Design review of the part built by this model. Coordinates are the model's own, in mm. Face numbers are marked on the shaded views. A direction names the side the tool comes from. Give positions to 0.01 mm unless a question says otherwise; leave off trailing zeros. Loops run counter-clockwise (first coordinate to the right, second up) from the corner with the lowest first, then second, coordinate; pieces in that order, holes last. Notation, with made-up numbers: M 8.25,8.25 L 39.25,8.25 A18 cw 39.25,34.25 Z; hole C 80,68 d7. An arc over 180 degrees is marked long. Use CSV: the item, a comma, the result in double quotes.
from build123d import *

# Parameters (mm, degrees)
F1_DEPTH = 31.75
F3_DEPTH = 2.032
F4_SIZE  = 5.08
F5_R     = 3.175
F6_DEPTH = 3.048
F7_R     = 1.5875
F9_DEPTH = 22.0939118459


with BuildPart() as f1:
    # F0 (on Top) → F1 (new body)
    with BuildSketch(Plane.XY):
        Polygon((-25.273, 19.05), (-25.273, 0), (25.273, 0), (25.273, 19.05), (44.45, 19.05), (44.45, 22.098), (22.225, 22.098), (22.225, 3.048), (-22.225, 3.048), (-22.225, 22.098), (-44.45, 22.098), (-44.45, 19.05), align=None)
    extrude(amount=F1_DEPTH)

    # F2 (on face) → F3 (join)
    with BuildSketch(Plane(origin=(0, 0, 0), x_dir=(1, 0, 0), z_dir=(0, 0, -1))):
        Polygon((25.273, 0), (-25.273, 0), (-25.273, -19.05), (-44.45, -19.05), (-44.45, -22.098), (-25.273, -22.098), (-6.35, -22.098), (-6.35, -18.923), (6.35, -18.923), (6.35, -22.098), (25.273, -22.098), (44.45, -22.098), (44.45, -19.05), (25.273, -19.05), align=None)
    extrude(amount=F3_DEPTH)

    # F4
    f4_edges = [f1.edges().sort_by_distance(p)[0] for p in [
        (44.45, 20.574, 31.75),
        (-44.45, 20.574, 31.75),
    ]]
    chamfer(f4_edges, length=F4_SIZE)

    # F5 (on face) → F6 (cut, through all)
    with BuildSketch(Plane.XZ.offset(-19.05)):
        with Locations((-34.8615, 12.319)):
            Circle(F5_R)
        with Locations((34.8615, 12.319)):
            Circle(F5_R)
    extrude(amount=-F6_DEPTH, mode=Mode.SUBTRACT)

    # F7
    f7_edges = [f1.edges().sort_by_distance(p)[0] for p in [
        (25.273, 0, 14.859),
        (-25.273, 0, 14.859),
        (25.273, 19.05, 14.859),
        (22.225, 3.048, 15.875),
        (22.225, 22.098, 15.875),
        (-22.225, 3.048, 15.875),
        (-22.225, 22.098, 15.875),
    ]]
    fillet(f7_edges, radius=F7_R)

    # F8 (on face) → F9 (cut, through all)
    with BuildSketch(Plane.XZ):
        Polygon((23.6855, 31.75), (-23.6855, 31.75), (0, 14.859), align=None)
    extrude(amount=-F9_DEPTH, mode=Mode.SUBTRACT)


solid = f1.part
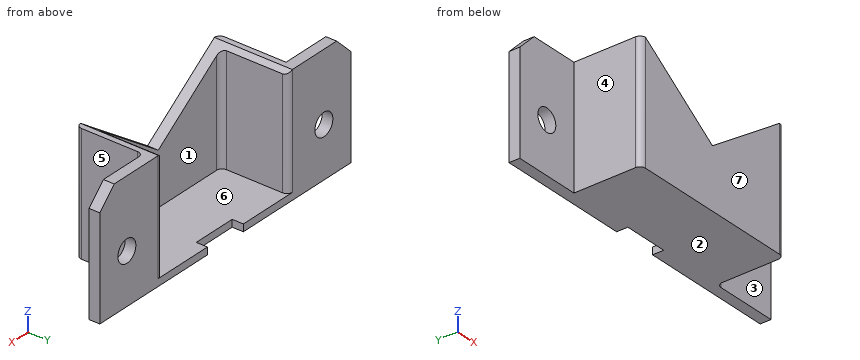
(1) Machinability: for the marked faces 1, 2, 3 and 4, which of the approach directions +Z, -Z, +X, -X, +Y, -Y give a long, thin tool a straight path to every point of the face, cutting with its end or side? Answer none if there is none.
A:
face 1,"+Z, +Y"
face 2,"-Z, +X, -X, +Y, -Y"
face 3,"+Z, -Z, +X, -Y"
face 4,"+Z, -Z, -X, -Y"
(2) Clearance check with flat-ended pins moving along their axes: P1, Ø1.6, axis at x = 2, z = -1.5, coming from the +Y side; P2, Ø12.5, axis at y = 10, z = 15, coming from the -X side; P3, Ø10, axis at x = 31, y = 5, coming from the -Z side; P4, Ø8, axis at x = -4.5, y = 2.5, coming from the +Z side. State where each tip first meets the part, or that it passes through.
A:
P1,"y = 18.92"
P2,"x = -25.27"
P3,"through"
P4,"z = 20.92"
(3) We need section B-B on z = 11.5. Count the separate pieces of the cut face and the enclosed holes in it, then the cut area to 3 significant figures.
A:
separate pieces,"3"
enclosed holes,"0"
area,"349 mm²"
(4) We need section A-A on x = -34. State the section outline as (y, z) points.
A:
outline,"M 19.05,-2.03 L 22.1,-2.03 L 22.1,9.26 L 19.05,9.26 Z; M 19.05,15.37 L 22.1,15.37 L 22.1,31.75 L 19.05,31.75 Z"
(5) Wall thickness on line 1 along X through (y, z) = (12.25, 7) (3 decimals); line 2 along Y through (x, z) = (-36.5, 29); line 3 along X through (y, z) = (18.5, 25.5) (3 decimals): over which ranges is each line inside the solid? List them lowest first. Write a range as [from, to].
A:
line 1,"[-25.273, -22.225], [22.225, 25.273]"
line 2,"[19.05, 22.1]"
line 3,"[-25.273, -22.225], [22.225, 25.659]"
(6) The part is to be moulded in two halves that separate along X. For the marked faces 5, 6 and 7, say which applies: released by +X, released by -X, zero draft, split by the parting line, or undercut.
A:
face 5,"released by +X"
face 6,"undercut"
face 7,"zero draft"
